Job drawing, mm, ordinate dimensions from the low corner. One solid piece. Round coordinates to 2 decimals unless told otherwise and drop trailing zeros. Write each loop counter-clockwise with the first axis right and the second up, starting at its lowest first coordinate (ties: lowest second). Pieces come first, ordered by that corner, then holes. Notation, with made-up numbers: M 6,-39 L 26,-39 A16 cw 26,-32 Z; hole C -1,30.25 d10. An arc over 180 degrees is marked long. Answer as a JSON object with one key per item and string values. Group by question number.
1. Band-saw the part on C-C, the plane z = 13. Write the cut outline in (x, y).
2. Band-saw the part on A-A, the plane x = 36.83. Count the separate pieces of the cut face and the enclosed holes in it.
3. Two-plate mould, pull along Y, no slides. Class the marked faces 1 and 2: +Y half, -Y half, draft (parallel to the pull), parting line (faces both ways), or undercut.
4. Drop flat-ended pins along their axis: pin 1 (2 mm diameter, centred on y = 49, z = 41.5, fed in from +X) (1 decimal); pin 2 (3 mm diameter, centred on y = 20, z = 90, fed in from +X); pin 3 (2 mm diameter, centred on x = 59.5, z = 44.5, fed in from -Y); pin 4 (1.5 mm diameter, centred on x = 36.83, z = 55.56, fed in from -Y). Give the stop position or say it passes through.
5. Drill centre lines: line 1 (X direction, y = 36.5, z = 81.5); line 2 (X direction, y = 36, z = 30). Where is each one in solid material? Low to high. Write a range as from..to.
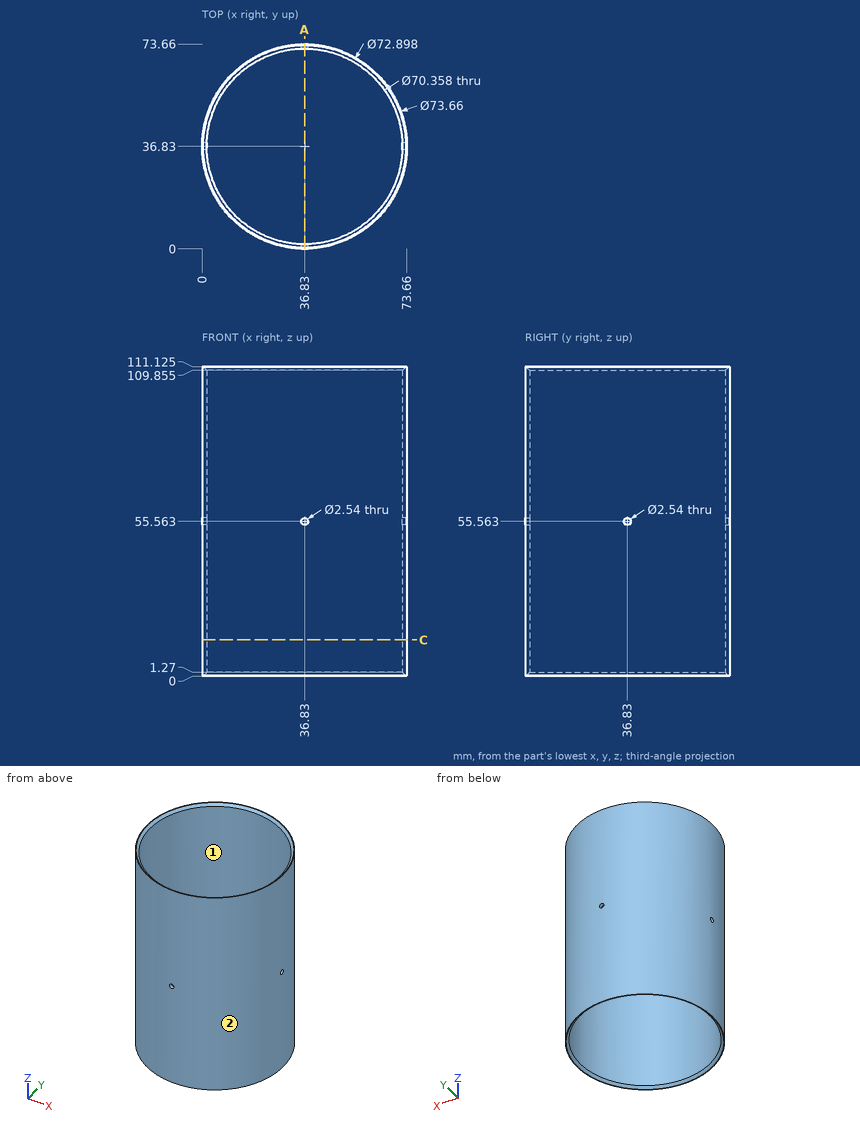
Worked answers:
{
 "1": {"outline": "C 36.83,36.83 d73.66; hole C 36.83,36.83 d70.36"},
 "2": {"separate pieces": "4", "enclosed holes": "0"},
 "3": {"face 1": "undercut", "face 2": "parting line"},
 "4": {"pin 1": "stops at x = 71.9", "pin 2": "stops at x = 70.32", "pin 3": "stops at y = 7.05", "pin 4": "passes through"},
 "5": {"line 1": "x = 0..1.65, 72.01..73.66", "line 2": "x = 0.01..1.66, 72..73.65"}
}
